from build123d import *

# Parameters (mm, degrees)
F1_DEPTH = 63.5
F0_W     = 26.9485112596
F0_H     = 19.05
F2_DEPTH = 25.4
F3_DEPTH = 9.2075
F4_R     = 6.35


with BuildPart() as f1:
    # F0 (on Front) → F1 (new body, symmetric)
    with BuildSketch(Plane.XZ):
        Polygon((-41.275, 9.525), (-41.275, -9.525), (41.275, -9.525), (41.275, 9.525), (22.225, 9.525), align=None)
    extrude(amount=F1_DEPTH, both=True)

    # F0 (on Front) → F2 (join, symmetric)
    with BuildSketch(Plane.XZ):
        with BuildLine():
            Line((22.225, 9.525), (41.275, 9.525))
            Line((41.275, 9.525), (41.275, 27.0002))
            ThreePointArc((41.275, 27.0002), (45.9246798487, 38.2255201513), (57.15, 42.8752))
            Line((57.15, 42.8752), (60.325, 42.8752))
            Line((60.325, 42.8752), (60.325, 61.9252))
            Line((60.325, 61.9252), (57.15, 61.9252))
            add(Edge.make_bspline(
                [(52.2492096808, 61.5796430153), (53.8592655061, 61.7142223816), (55.4926449754, 61.8294562532), (57.15, 61.9252)],
                knots=[107.5950176297, 107.5950176297, 107.5950176297, 107.5950176297, 111.5045361635, 111.5045361635, 111.5045361635, 111.5045361635], degree=3))
            ThreePointArc((52.2492096808, 61.5796430153), (30.7784649015, 49.8977492477), (22.225, 27.0002))
            Line((22.225, 27.0002), (22.225, 9.525))
        make_face()
        with Locations((73.7992556298, 52.4002)):
            Rectangle(F0_W, F0_H)
    extrude(amount=F2_DEPTH, both=True)

    # F0 (on Front) → F3 (join, symmetric)
    with BuildSketch(Plane.XZ):
        with BuildLine():
            add(Edge.make_bspline(
                [(-41.275, 9.525), (-18.7066018439, 39.5193474562), (7.9383863878, 57.8758444109), (52.2492096808, 61.5796430153)],
                knots=[0, 0, 0, 0, 107.5950176297, 107.5950176297, 107.5950176297, 107.5950176297], degree=3))
            Line((-41.275, 9.525), (22.225, 9.525))
            Line((22.225, 9.525), (22.225, 27.0002))
            ThreePointArc((22.225, 27.0002), (30.7784649015, 49.8977492477), (52.2492096808, 61.5796430153))
        make_face()
    extrude(amount=F3_DEPTH, both=True)

    # F4
    f4_edges = [f1.edges().sort_by_distance(p)[0] for p in [
        (-41.275, -63.5, 0),
        (41.275, -63.5, 0),
        (41.275, 63.5, 0),
        (-41.275, 63.5, 0),
    ]]
    fillet(f4_edges, radius=F4_R)

    # F0 (on Front) → F5 (revolve)
    with BuildSketch(Plane.XZ):
        Polygon((60.325, 66.675), (60.325, 61.9252), (87.2735112596, 61.9252), (87.2735112596, 42.8752), (60.325, 42.8752), (60.325, 38.1), (111.125, 38.1), (111.125, 66.675), align=None)
    revolve(axis=Axis((60.325, 0, 52.3875), (0, 0, 1)))


solid = f1.part
For this review, take the finished solid that the model builds, in its own axes (mm). A direction names the side the tool comes from. Coordinates: 2 decimals unless noted, no trailing zeros. Loops run counter-clockwise (first coordinate to the right, second up) from the corner with the lowest first, then second, coordinate; pieces in that order, holes last. Notation, with made-up numbers: (-28.75, 46) - (-10.75, 46) arc R12 cw to (-10.75, 69) - close; hole circle Ø3 at (-11, 31). An arc over 180 degrees is marked (long way). Return JSON: item names as keys, results as strings.
Item 1: Take a section at D-D (y = 53.5). Give the boundary of the cut face in (x, z) (3 decimals).
Determined:
{"outline": "(-41.275, -9.525) - (41.275, -9.525) - (41.275, 9.525) - (-41.275, 9.525) - close"}
Item 2: Take a section at B-B (x = 64). Give the boundary of the cut face in (y, z) (3 decimals).
Determined:
{"outline": "(-50.667, 38.1) - (50.667, 38.1) - (50.667, 66.675) - (-50.667, 66.675) - close; hole (-26.697, 42.875) - (-25.4, 42.875) - (-25.4, 61.925) - (-26.697, 61.925) - close; hole (25.4, 42.875) - (26.697, 42.875) - (26.697, 61.925) - (25.4, 61.925) - close"}
Item 3: For faces 4 (the flat face through (41.275, -1, 4)), 5 (the cylindrical face through (45.194, -15.618, 59.815)), 6 (the flat face through (31, 25.4, 24)), list the 3-axis set-ups (+Z, -Z, +X, -X, +Y, -Y) from which the entire face can be reached by the end or side of a thin tool; tool diameter is ignored.
Determined:
{"face 4": "-Z, +X, +Y, -Y", "face 5": "none", "face 6": "+X, -X, +Y"}
Item 4: Mouldability with a two-part tool opening along X and no side actions: class faces 1 (the flat face through (22.225, 17, 18)), 2 (the flat face through (40, -9.208, 59)), 3 (the flat face through (31, -25.4, 24)) as pulls with the +X half, pulls with the -X half, needs draft (parallel to the pull), parting line crosses it, or undercut.
Determined:
{"face 1": "pulls with the -X half", "face 2": "undercut", "face 3": "needs draft"}
Item 5: Take a section at C-C (y = 36.5). Give the boundary of the cut face in (x, z) (3 decimals), then the cut area to 3 significant figures.
Determined:
{"outline": "(-41.275, -9.525) - (41.275, -9.525) - (41.275, 9.525) - (-41.275, 9.525) - close; (24.992, 38.1) - (95.658, 38.1) - (95.658, 66.675) - (24.992, 66.675) - close", "area": "3,590 mm2"}
Item 6: Insertion check: pin 1 (2.5 mm diameter, centred on x = 39.5, z = 57, fed in from -Y); pin 2 (2 mm diameter, centred on x = -22, z = 27, fed in from -Y); pin 3 (1 mm diameter, centred on y = -31, z = 39.5, fed in from -X). Each pin has a flat end and moves straight along its axis. Give the tip position at first contact, or say it passes through.
Determined:
{"pin 1": "stops at y = -46.88", "pin 2": "stops at y = -9.21", "pin 3": "stops at x = 19.7"}
Item 7: Take a section at A-A (y = -42.5). Give the boundary of the cut face in (x, z) (3 decimals), then the cut area to 3 significant figures.
Determined:
{"outline": "(-41.275, -9.525) - (41.275, -9.525) - (41.275, 9.525) - (-41.275, 9.525) - close; (32.497, 38.1) - (88.153, 38.1) - (88.153, 66.675) - (32.497, 66.675) - close", "area": "3,160 mm2"}
Item 8: For line 1 (Y direction, x = 56, z = 56); line 2 (Z direction, x = 12, y = 16) (3 decimals); line 3 (Y direction, x = 2, z = 28), list the stretches that pass through material, from the lowest coordinate up.
Determined:
{"line 1": "y = -50.62 to -26.6, -25.4 to 25.4, 26.6 to 50.62", "line 2": "z = -9.525 to 9.525", "line 3": "y = -9.21 to 9.21"}
